The drawing under review shows one solid part. Ordinate dimensions are in mm from its lowest x, y, z. A direction names the side the tool comes from. Coordinates: 2 decimals unless noted, no trailing zeros. Write each loop counter-clockwise with the first axis right and the second up, starting at its lowest first coordinate (ties: lowest second). Pieces come first, ordered by that corner, then holes.
1) Add section B-B, the plane z = 8. State the section outline as (x, y) points.
2) For line 1 (Z direction, x = 16.5, y = 12); line 2 (X direction, y = 1.25, z = 36), list the stretches that pass through material, from the lowest coordinate up.
3) Machinability: for the marked faces 1, 2 and 3, which of the approach directions +Z, -Z, +X, -X, +Y, -Y give a long, thin tool a straight path to every point of the face, cutting with its end or side? Answer none if there is none.
4) Add section A-A, the plane z = 30.5. State the section outline as (x, y) points.
5) For P1, Ø16, axis at x = 10, z = 52, coming from the -Y side; P2, Ø6.5, axis at x = 13.5, y = 10.5, coming from the +Z side; P3, Ø3, axis at x = 330, y = 10.5, coming from the -Z side, all flat-tipped, find the tip position at first contact; note any pin that passes through.
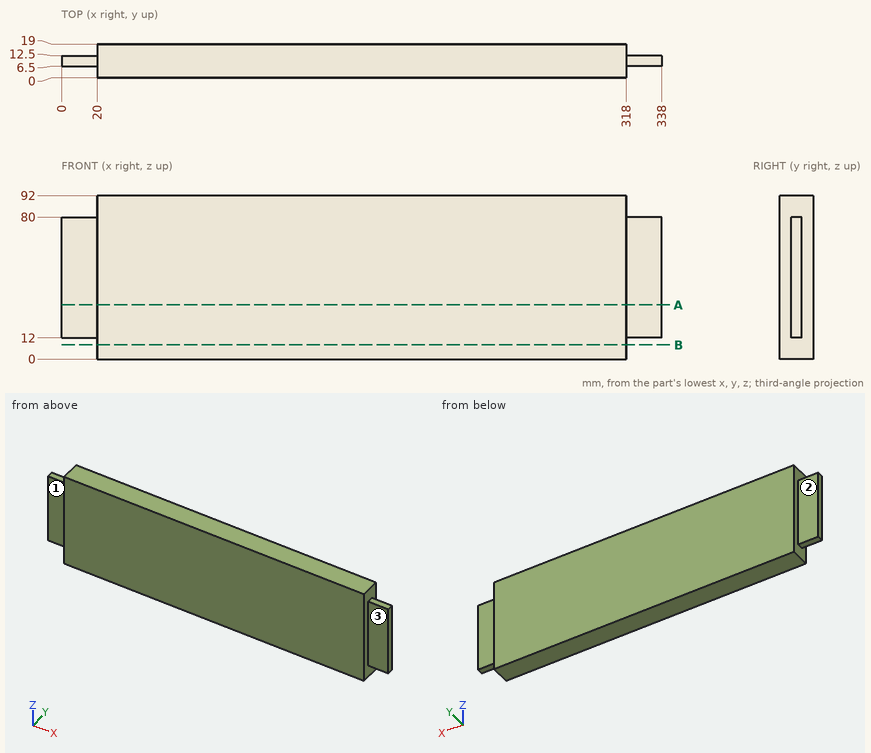
Geometry results:
1. outline: (20, 0) - (318, 0) - (318, 19) - (20, 19) - close
2. line 1: z = 12 to 80
2. line 2: x = 20 to 318
3. face 1: +Z, -Z, -X, -Y
3. face 2: +Z, -Z, -X, +Y
3. face 3: +Z, -Z, +X, -Y
4. outline: (0, 6.5) - (20, 6.5) - (20, 0) - (318, 0) - (318, 6.5) - (338, 6.5) - (338, 12.5) - (318, 12.5) - (318, 19) - (20, 19) - (20, 12.5) - (0, 12.5) - close
5. P1: stops at y = 6.5
5. P2: stops at z = 80
5. P3: stops at z = 12
